from build123d import *

# Parameters (mm, degrees)
F1_DEPTH      = 36.068
F1_DEPTH_BACK = 36.068
F3_DEPTH      = 33.274
F3_DEPTH_BACK = 34.036


with BuildPart() as f1:
    # F0 (on Right) → F1 (new body, two sides)
    with BuildSketch(Plane.YZ) as f1_sk:
        with BuildLine():
            Line((67.711897, 0), (53.822275, 0))
            Line((53.822275, 0), (-53.822279, 0))
            ThreePointArc((-53.822279, 0), (-60.71707, 17.182161), (-42.39228, 19.821646))
            Line((-42.39228, 19.821646), (-39.498609, 23.294052))
            ThreePointArc((-39.498609, 23.294052), (-65.444359, 18.845353), (-53.822279, -4.774557))
            Line((-53.822279, -4.774557), (67.711897, -4.774557))
            Line((67.711897, -4.774557), (67.711897, 0))
        make_face()
    extrude(amount=F1_DEPTH)
    extrude(f1_sk.sketch, amount=-F1_DEPTH_BACK)

    # F2 (on Right) → F3 (join, two sides)
    with BuildSketch(Plane.YZ) as f3_sk:
        with BuildLine():
            Line((-20.712223, 20.559708), (-20.712223, 0))
            Line((-20.712223, 0), (63.800037, 0))
            Line((63.800037, 0), (63.800037, 34.184899))
            Line((63.800037, 34.184899), (40.267568, 34.184899))
            Line((40.267568, 34.184899), (40.267568, 12.495875))
            Line((40.267568, 12.495875), (16.530469, 12.495875))
            Line((16.530469, 12.495875), (16.530469, 34.184899))
            Line((16.530469, 34.184899), (-10.077052, 34.184899))
            ThreePointArc((-10.077052, 34.184899), (-18.609421, 29.881609), (-20.712223, 20.559708))
        make_face()
    extrude(amount=F3_DEPTH)
    extrude(f3_sk.sketch, amount=-F3_DEPTH_BACK)


solid = f1.part
The model under review builds one solid part; all positions refer to its coordinate system, in mm. A direction names the side the tool comes from. Coordinates: 2 decimals unless noted, no trailing zeros. Write each loop counter-clockwise with the first axis right and the second up, starting at its lowest first coordinate (ties: lowest second). Pieces come first, ordered by that corner, then holes. Notation, with made-up numbers: (-9, 23.5) -> (28, 23.5) arc R15 cw to (28, 29.5) -> close; hole circle Ø3 at (19, -37.5). An arc over 180 degrees is marked (long way). Answer in a Markdown table with one row per item.
1. Clearance check with flat-ended pins moving along their axes: pin 1 Ø1 at (x, z) = (13, 22) entering from -Y; pin 2 Ø3 at (y, z) = (1.5, 4.5) entering from +X; pin 3 Ø11 at (x, z) = (-12, 28) entering from +Y; pin 4 Ø16.5 at (x, z) = (-16, 11.5) entering from -Y. State where each tip first meets the part, or that it passes through.
Answers below:
| item | result |
|---|---|
| pin 1 | stops at y = -63.75 |
| pin 2 | stops at x = 33.27 |
| pin 3 | stops at y = 63.8 |
| pin 4 | stops at y = -67.24 |
2. We need section A-A, the plane y = 13.5. State the section outline as (x, z) points.
Answers below:
| item | result |
|---|---|
| outline | (-36.07, -4.77) -> (36.07, -4.77) -> (36.07, 0) -> (33.27, 0) -> (33.27, 34.18) -> (-34.04, 34.18) -> (-34.04, 0) -> (-36.07, 0) -> close |
3. For faces 1 (the flat face through (0, -20.712, 10)), 2 (the flat face through (-1, 63.8, 17)), 3 (the flat face through (0, 40.268, 23)), 4 (the flat face through (-34.036, 21, 10)), 5 (the flat face through (-36.068, -15.1, -0.5)), list the 3-axis set-ups (+Z, -Z, +X, -X, +Y, -Y) from which the entire face can be reached by the end or side of a thin tool; tool diameter is ignored.
Answers below:
| item | result |
|---|---|
| face 1 | +X, -X |
| face 2 | +Z, +X, -X, +Y |
| face 3 | +Z, +X, -X |
| face 4 | +Z, -X, +Y |
| face 5 | +Z, -Z, -X, +Y, -Y |
4. We need section D-D, the plane z = 26. State the section outline as (x, y) points.
Answers below:
| item | result |
|---|---|
| outline | (-36.07, -58.3) -> (36.07, -58.3) -> (36.07, -43.32) -> (-36.07, -43.32) -> close; (-34.04, -20.57) -> (33.27, -20.57) -> (33.27, 16.53) -> (-34.04, 16.53) -> close; (-34.04, 40.27) -> (33.27, 40.27) -> (33.27, 63.8) -> (-34.04, 63.8) -> close |
5. Draft analysis for pull direction Y (two halves, no side actions). For faces 6 (the cylindrical face through (0.505, -60.863, 16.922)), 7 (the flat face through (33.274, 21, 10)), 8 (the flat face through (1, 67.712, -2)), state which applies: +Y half, -Y half, draft (parallel to the pull), parting line (faces both ways), or undercut.
Answers below:
| item | result |
|---|---|
| face 6 | undercut |
| face 7 | draft |
| face 8 | +Y half |
6. We need section B-B, the plane z = 1.5. State the section outline as (x, y) points, and give its area (3 significant figures).
Answers below:
| item | result |
|---|---|
| outline | (-36.07, -63.94) -> (36.07, -63.94) -> (36.07, -57.04) -> (-36.07, -57.04) -> close; (-34.04, -20.71) -> (33.27, -20.71) -> (33.27, 63.8) -> (-34.04, 63.8) -> close |
| area | 6,190 mm^2 |
7. We need section C-C, the plane x = -16. State the section outline as (y, z) points, and give its area (3 significant figures).
Answers below:
| item | result |
|---|---|
| outline | (-53.82, -4.77) -> (67.71, -4.77) -> (67.71, 0) -> (63.8, 0) -> (63.8, 34.18) -> (40.27, 34.18) -> (40.27, 12.5) -> (16.53, 12.5) -> (16.53, 34.18) -> (-10.08, 34.18) arc R11.2 ccw to (-20.71, 20.56) -> (-20.71, 0) -> (-53.82, 0) arc R11.77 cw (long way) to (-42.39, 19.82) -> (-39.5, 23.29) arc R16.43 ccw (long way) to start |
| area | 3,180 mm^2 |
8. Wall thickness on probe 1 along Y at (x, z) = (16, 26); probe 2 along Y at (x, z) = (-4, 13); probe 3 along X at (y, z) = (-1, 24): over which ranges is each line inside the solid? List them lowest first. Write a range as [from, to].
Answers below:
| item | result |
|---|---|
| probe 1 | y = [-58.3, -43.32], [-20.57, 16.53], [40.27, 63.8] |
| probe 2 | y = [-67.16, -62.17], [-20.71, 16.53], [40.27, 63.8] |
| probe 3 | x = [-34.04, 33.27] |
